from build123d import *

# Parameters (mm, degrees)
SKETCH1_W           = 405
SKETCH1_H           = 130
BOSS_EXTRUDE1_DEPTH = 5
SKETCH2_W           = 5
SKETCH2_H           = 60
CUT_EXTRUDE1_DEPTH  = 5
SKETCH3_W           = 5
SKETCH3_H           = 20
CUT_EXTRUDE2_DEPTH  = 10
SKETCH4_W           = 20
SKETCH4_H           = 5
CUT_EXTRUDE3_DEPTH  = 10
SKETCH5_R           = 7.5
CUT_EXTRUDE4_DEPTH  = 10


with BuildPart() as part:
    # Sketch1 → Boss-Extrude1 (new body)
    with BuildSketch(Plane.XY):
        with Locations((-202.5, -65)):
            Rectangle(SKETCH1_W, SKETCH1_H)
    extrude(amount=BOSS_EXTRUDE1_DEPTH)

    # Sketch2 → Cut-Extrude1 (cut)
    with BuildSketch(Plane(origin=(0, 0, 0), x_dir=(-1, 0, 0), z_dir=(0, 0, -1))):
        with Locations((402.5, -65)):
            Rectangle(SKETCH2_W, SKETCH2_H)
        with Locations((2.5, -65)):
            Rectangle(SKETCH2_W, SKETCH2_H)
    extrude(amount=-CUT_EXTRUDE1_DEPTH, mode=Mode.SUBTRACT)

    # Sketch3 → Cut-Extrude2 (cut)
    with BuildSketch(Plane.XY.offset(5)):
        with Locations((-392.5, -110)):
            Rectangle(SKETCH3_W, SKETCH3_H)
        with Locations((-392.5, -50)):
            Rectangle(SKETCH3_W, SKETCH3_H)
        with Locations((-352.5, -50)):
            Rectangle(SKETCH3_W, SKETCH3_H)
        with Locations((-352.5, -110)):
            Rectangle(SKETCH3_W, SKETCH3_H)
        with Locations((-52.5, -110)):
            Rectangle(SKETCH3_W, SKETCH3_H)
        with Locations((-52.5, -50)):
            Rectangle(SKETCH3_W, SKETCH3_H)
        with Locations((-12.5, -50)):
            Rectangle(SKETCH3_W, SKETCH3_H)
        with Locations((-12.5, -110)):
            Rectangle(SKETCH3_W, SKETCH3_H)
    extrude(amount=-CUT_EXTRUDE2_DEPTH, mode=Mode.SUBTRACT)

    # Sketch4 → Cut-Extrude3 (cut)
    with BuildSketch(Plane.XY.offset(5)):
        with Locations((-372.5, -112.5)):
            Rectangle(SKETCH4_W, SKETCH4_H)
        with Locations((-372.5, -72.5)):
            Rectangle(SKETCH4_W, SKETCH4_H)
        with Locations((-32.5, -112.5)):
            Rectangle(SKETCH4_W, SKETCH4_H)
        with Locations((-32.5, -72.5)):
            Rectangle(SKETCH4_W, SKETCH4_H)
    extrude(amount=-CUT_EXTRUDE3_DEPTH, mode=Mode.SUBTRACT)

    # Sketch5 → Cut-Extrude4 (cut)
    with BuildSketch(Plane.XY.offset(5)):
        with Locations((-372.5, -92.5)):
            Circle(SKETCH5_R)
        with Locations(Location((-32.5, -92.5, 0), (0, 0, 180))):
            Circle(SKETCH5_R)
    extrude(amount=-CUT_EXTRUDE4_DEPTH, mode=Mode.SUBTRACT)


solid = part.part
CAD build for the part. Positions are in the model's coordinates, mm. Give positions to 0.01 mm unless a question says otherwise; leave off trailing zeros. Order: outer loops, then holes, each group sorted by start corner. A loop starts at its lowest first (then second) coordinate and runs counter-clockwise, first axis right, second up. Notation, with made-up numbers: (25, 40.5) - (40, 40.5) arc R17 cw to (40, 69.5) - close; hole circle Ø6 at (52.25, 85). An arc over 180 degrees is marked (long way). Answer in a Markdown table with one row per item.
1. Saw through at A-A, the plane x = -32.5. Give the cut face in (y, z).
Data:
| item | result |
|---|---|
| outline | (-130, 0) - (-115, 0) - (-115, 5) - (-130, 5) - close; (-110, 0) - (-100, 0) - (-100, 5) - (-110, 5) - close; (-85, 0) - (-75, 0) - (-75, 5) - (-85, 5) - close; (-70, 0) - (0, 0) - (0, 5) - (-70, 5) - close |
2. Probe probe 1 along Y at (x, z) = (-32.5, 1.8); probe 2 along X at (y, z) = (-43, 3.65); probe 3 along X at (y, z) = (-72, 1.65). List the from-to ranges inside material, lowest first. Write a range as [from, to].
Data:
| item | result |
|---|---|
| probe 1 | y = [-130, -115], [-110, -100], [-85, -75], [-70, 0] |
| probe 2 | x = [-400, -395], [-390, -355], [-350, -55], [-50, -15], [-10, -5] |
| probe 3 | x = [-400, -382.5], [-362.5, -42.5], [-22.5, -5] |
3. Flat gauge pin, fed straight in: pin 1 (2.5 mm diameter, centred on y = -53, z = 2, fed in from +X). Where does the tip first touch, or does it go through?
Data:
| item | result |
|---|---|
| pin 1 | stops at x = -5 |
4. Pull direction Y, two halves, no side cores. Call faces 1 (the flat face through (-205, -64, 5)), 2 (the cylindrical face through (-365.57, -95.37, 2.54)), 3 (the cylindrical face through (-30.87, -85.18, 2.54)): pulls with the +Y half, pulls with the -Y half, needs draft (parallel to the pull), parting line crosses it, or undercut.
Data:
| item | result |
|---|---|
| face 1 | needs draft |
| face 2 | undercut |
| face 3 | undercut |
5. Saw through at C-C, the plane y = -79. Give the cut face in (x, z), plus the area to 4 significant figures.
Data:
| item | result |
|---|---|
| outline | (-400, 0) - (-5, 0) - (-5, 5) - (-400, 5) - close |
| area | 1,975 mm² |
6. Saw through at B-B, the plane z = 1.15. Count the separate pieces of the cut face and the enclosed holes in it, plus the area to 3 significant figures.
Data:
| item | result |
|---|---|
| separate pieces | 1 |
| enclosed holes | 14 |
| area | 50,500 mm² |
